```python
from build123d import *

# Parameters (mm, degrees)
F3_DEPTH = 0.5


with BuildPart() as f3:
    # F2 (on Front) → F3 (new body, symmetric)
    with BuildSketch(Plane.XZ):
        Polygon((-16, 0), (-17, 0), (-17, -1), (-18, -1), (-18.9205025733, -0.2568606869), (-18.9205025733, 0.4893779857), (-19.9205025733, 0.4893779857), (-19.9205025733, -1.0106220143), (-18, -2.5), (-17, -2.5), (-16, -2.5), (-15, -1.4226497308), (-15, -0.4226497308), (-16, -1), align=None)
    extrude(amount=F3_DEPTH, both=True)



with BuildPart() as f3b:
    # F2 (on Front) → F3, piece 2 (new body, symmetric)
    with BuildSketch(Plane.XZ):
        Polygon((17, 0), (16, 0), (16, -1), (15, -0.4226497308), (15, -1.4226497308), (16, -2.5), (17, -2.5), (18, -2.5), (19.9205025733, -1.0106220143), (19.9205025733, 0.4893779857), (18.9205025733, 0.4893779857), (18.9205025733, -0.2568606869), (18, -1), (17, -1), align=None)
    extrude(amount=F3_DEPTH, both=True)


with BuildPart() as f3_1:
    add(f3.part)

    add(f3b.part)  # F4 merges F3b
    # F4: sweep along a path in F0
    with BuildLine(Plane.XY) as f4_path:
        ThreePointArc((-16, -0.5), (0, -16.5), (16, -0.5))
        Line((16, -0.5), (16, 0.5))
        ThreePointArc((16, 0.5), (0, 16.5), (-16, 0.5))
        Line((-16, 0.5), (-16, -0.5))
    # F1 (on Front) → F4 (sweep)
    with BuildSketch(Plane.XZ):
        Polygon((16, 0), (18, 0), (18, 1.5), (21, 1.5), (21, 2.5), (20.5, 2.5), (20.5, 3.5), (21, 3.5), (21, 4.5), (19, 4.5), (19, 3.2320508076), (16, 1.5), align=None)
    sweep(path=f4_path.line)


solid = f3_1.part
```
Model file for the job. Use its own axes, mm. A direction names the side the tool comes from. Round coordinates to 2 decimals unless told otherwise and drop trailing zeros. Write each loop counter-clockwise with the first axis right and the second up, starting at its lowest first coordinate (ties: lowest second). Pieces come first, ordered by that corner, then holes. Notation, with made-up numbers: M 68,14 L 95,14 A5 cw 95,23 Z; hole C 28.25,-21.5 d11. An arc over 180 degrees is marked long. Put each result on its own line as item: value.
Item 1: Mould opens along X. For faces 6 (the flat face through (-21, 0, 4)), 7 (the flat face through (-19.4, 0, 0.489)), 8 (the flat face through (15.507, -0.007, -0.715)) say: +X half, -X half, draft (parallel to the pull), parting line (faces both ways), or undercut.
Responses:
face 6: -X half
face 7: draft
face 8: undercut
Item 2: Probe L1, parallel to Y at x = -1, z = 3; L2, parallel to X at y = 5, z = 2; L3, parallel to X at y = -10, z = 2. List the from-to ranges inside material, lowest first. Write a range as from..to.
Responses:
L1: -20.98..-19.07, 19.07..20.98
L2: -20.51..-16.25, 16.25..20.51
L3: -18.73..-13.94, 13.94..18.73
Item 3: Flat gauge pins, fed straight in: P1, Ø1, axis at y = 12, z = -1, coming from the +X side (3 decimals); P2, Ø0.5, axis at y = 0, z = 0, coming from the -X side; P3, Ø10, axis at x = 5, y = -11.5, coming from the +Z side; P4, Ø0.5, axis at y = 0, z = -1, coming from the +X side. Where does each tip first touch, or does it go through?
Responses:
P1: through
P2: x = -19.92
P3: z = 2.13
P4: x = 19.92
Item 4: Tool access for faces 1 (the cylindrical face through (0.352, 16.496, 0.74)), 2 (the flat face through (17, 0, -0.5)), 3 (the cylindrical face through (0, 21, 3)), 4 (the flat face through (-20.5, 0, 3)), 5 (the cylindrical face through (0.418, 19.495, 3.857)): list every direction of +Z, -Z, +X, -X, +Y, -Y with a clear straight run to the whole face (end or side of a thin tool).
Responses:
face 1: +Z, -Z
face 2: +Y, -Y
face 3: +Y
face 4: -X, +Y, -Y
face 5: +Z
Item 5: Cut at C-C (z = 2). List the corners of the cut face in (x, y).
Responses:
outline: M -21,-0.5 A21 ccw 21,-0.5 L 21,0.5 A21 ccw -21,0.5 Z; hole M -16.87,-0.5 A16.87 ccw 16.87,-0.5 L 16.87,0.5 A16.87 ccw -16.87,0.5 Z
Item 6: Cut at A-A (x = 0). List the corners of the cut face in (y, z), and give its area (3 significant figures).
Responses:
outline: M -21.5,1.5 L -18.5,1.5 L -18.5,0 L -16.5,0 L -16.5,1.5 L -19.5,3.23 L -19.5,4.5 L -21.5,4.5 L -21.5,3.5 L -21,3.5 L -21,2.5 L -21.5,2.5 Z; M 16.5,0 L 18.5,0 L 18.5,1.5 L 21.5,1.5 L 21.5,2.5 L 21,2.5 L 21,3.5 L 21.5,3.5 L 21.5,4.5 L 19.5,4.5 L 19.5,3.23 L 16.5,1.5 Z
area: 22.2 mm²
Item 7: Cut at B-B (z = -2). List the corners of the cut face in (x, y), and give its area (3 significant figures).
Responses:
outline: M -18.64,-0.5 L -15.54,-0.5 L -15.54,0.5 L -18.64,0.5 Z; M 15.54,-0.5 L 18.64,-0.5 L 18.64,0.5 L 15.54,0.5 Z
area: 6.22 mm²
